Print and shaded views of the part. All mm, measured from the part's lowest x, y and z. A direction names the side the tool comes from. Give positions to 0.01 mm unless a question says otherwise; leave off trailing zeros. Write each loop counter-clockwise with the first axis right and the second up, starting at its lowest first coordinate (ties: lowest second). Pieces come first, ordered by that corner, then holes. Notation, with made-up numbers: M 8,-3.5 L 39,-3.5 A27 ccw 39,35.5 Z; hole C 78,15 d7. An arc over 180 degrees is marked long. One line per question, with ' | ' between items. Start each with the question number.
1. Wall check: L1, parallel to Z at x = 57, y = 10.25; L2, parallel to X at y = 19.5, z = 57.5. Give the ranges that are in metal, low to high.
2. Pull direction Z, two halves, no side cores. Call the marked faces 1, 2, 3 and 4: released by +Z, released by -Z, zero draft, split by the parting line, or undercut.
3. Cut at A-A, the plane x = 7.5. Write the cut outline in (y, z).
4. Cut at B-B, the plane z = 27.5. Write the cut outline in (x, y).
5. Cut at C-C, the plane y = 21.25. Write the cut outline in (x, z).
6. Which spindle directions (+Z, -Z, +X, -X, +Y, -Y) get a long thin tool onto all of the face, cutting with end or side? Do the marked faces 5 and 6. Say none if no direction does.
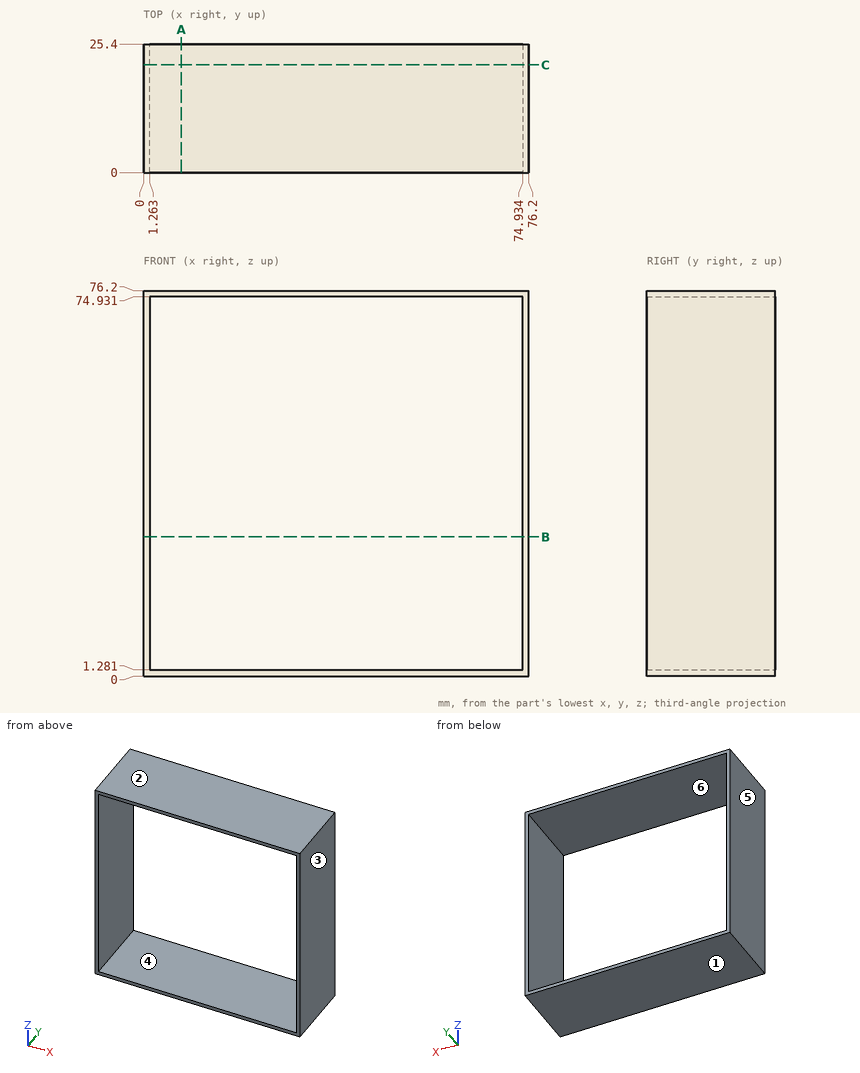
Here are the results:
1) L1: 0 to 1.28, 74.93 to 76.2 | L2: 0 to 1.26, 74.93 to 76.2
2) face 1: released by -Z | face 2: released by +Z | face 3: zero draft | face 4: undercut
3) outline: M 0,0 L 25.4,0 L 25.4,1.28 L 0,1.28 Z; M 0,74.93 L 25.4,74.93 L 25.4,76.2 L 0,76.2 Z
4) outline: M 0,0 L 1.26,0 L 1.26,25.4 L 0,25.4 Z; M 74.93,0 L 76.2,0 L 76.2,25.4 L 74.93,25.4 Z
5) outline: M 0,0 L 76.2,0 L 76.2,76.2 L 0,76.2 Z; hole M 1.26,1.28 L 74.93,1.28 L 74.93,74.93 L 1.26,74.93 Z
6) face 5: +Z, -Z, -X, +Y, -Y | face 6: +Y, -Y
